```python
from build123d import *

# Parameters (mm, degrees)
F0_W     = 63.5
F0_H     = 127
F0_W_2   = 58.42
F0_H_2   = 121.92
F0_W_3   = 9.398
F0_H_3   = 9.398
F0_W_4   = 12.7
F0_H_4   = 37.084
F0_W_5   = 51.054
F0_H_5   = 21.59
F1_DEPTH = 2.54
F2_DEPTH = 38.1
F3_W     = 58.42
F3_H     = 2.54
F4_DEPTH = 2.54
F6_DEPTH = 12.0904


with BuildPart() as f1:
    # F0 (on Front) → F1 (new body)
    with BuildSketch(Plane.XZ):
        Rectangle(F0_W, F0_H)
        Rectangle(F0_W_2, F0_H_2, mode=Mode.SUBTRACT)
        Rectangle(F0_W_2, F0_H_2)
        with Locations((-19.05, -4.699)):
            Rectangle(F0_W_3, F0_H_3, mode=Mode.SUBTRACT)
        with Locations((19.05, -16.002)):
            Rectangle(F0_W_4, F0_H_4, mode=Mode.SUBTRACT)
        with Locations((0, 40.005)):
            Rectangle(F0_W_5, F0_H_5, mode=Mode.SUBTRACT)
    extrude(amount=-F1_DEPTH)

    # F0 (on Front) → F2 (join)
    with BuildSketch(Plane.XZ):
        Rectangle(F0_W, F0_H)
        Rectangle(F0_W_2, F0_H_2, mode=Mode.SUBTRACT)
    extrude(amount=-F2_DEPTH)

    # F3 (on face) → F4 (join)
    with BuildSketch(Plane(origin=(0, 0, 60.96), x_dir=(1, 0, 0), z_dir=(0, 0, -1))):
        with Locations((0, -36.83)):
            Rectangle(F3_W, F3_H)
    extrude(amount=F4_DEPTH)

    # F5 (on face) → F6 (cut)
    with BuildSketch(Plane.XY.offset(63.5)):
        with BuildLine():
            ThreePointArc((-23.5712, 27.7114), (-18.4912, 22.6314), (-13.4112, 27.7114))
            ThreePointArc((-13.4112, 27.7114), (-18.4912, 32.7914), (-23.5712, 27.7114))
        make_face()
        with BuildLine():
            ThreePointArc((-23.5712, 27.7114), (-18.4912, 32.7914), (-13.4112, 27.7114))
            Line((-13.4112, 27.7114), (-13.4112, 38.1))
            Line((-13.4112, 38.1), (-23.5712, 38.1))
            Line((-23.5712, 38.1), (-23.5712, 27.7114))
        make_face()
    extrude(amount=-F6_DEPTH, mode=Mode.SUBTRACT)


solid = f1.part
```
Geometry: final body of the model. Coordinates: model frame, mm. A direction names the side the tool comes from. Round coordinates to 2 decimals unless told otherwise and drop trailing zeros. Write each loop counter-clockwise with the first axis right and the second up, starting at its lowest first coordinate (ties: lowest second). Pieces come first, ordered by that corner, then holes.
Item 1: Section query B-B (y = 13). Return loops of the section in (x, z), plus the area to 3 significant figures.
Item 2: Mould query, pull axis X, two halves, no side actions, for faces 5 (the face through (8, 37, 58.42)), 6 (the face through (31.75, 19, -1)), 7 (the face through (-31.75, 19, -1)). Classes: +X half, -X half, draft (parallel to the pull), parting line (faces both ways), or undercut.
Item 3: Section query D-D (z = -29). Return loops of the section in (x, y).
Item 4: Pin query (flat end, axial travel): P1, Ø3, axis at x = -19, z = 28.5, coming from the +Y side; P2, Ø12, axis at x = -22, z = -49.5, coming from the -Y side. Return the tip coordinate at first contact, or that it passes through.
Item 5: Section query C-C (x = 23.5). Return loops of the section in (y, z), plus the area to 3 significant figures.
Item 6: Section query A-A (x = -8.5). Return loops of the section in (y, z).
Item 7: Material intervals for L1, parallel to Z at x = 21, y = 4; L2, parallel to X at y = 32, z = -12; L3, parallel to Y at x = -4, z = -34, sorted ascending.
Item 8: Set-up query: faces 1 (the face through (-26, 35.56, 60)), 2 (the face through (-26, 37, 58.42)), 3 (the face through (-19, 1, 0)), 4 (the face through (-13.411, 34, 62)). Return all of +Z, -Z, +X, -X, +Y, -Y with unobstructed straight access to the full face (end or side cutting, diameter ignored); none if empty.
Completed:
1. outline: (-31.75, -63.5) - (31.75, -63.5) - (31.75, 63.5) - (-31.75, 63.5) - close; hole (-29.21, -60.96) - (29.21, -60.96) - (29.21, 60.96) - (-29.21, 60.96) - close
1. area: 942 mm2
2. face 5: undercut
2. face 6: +X half
2. face 7: -X half
3. outline: (-31.75, 0) - (12.7, 0) - (12.7, 2.54) - (-29.21, 2.54) - (-29.21, 38.1) - (-31.75, 38.1) - close; (25.4, 0) - (31.75, 0) - (31.75, 38.1) - (29.21, 38.1) - (29.21, 2.54) - (25.4, 2.54) - close
4. P1: stops at y = 2.54
4. P2: stops at y = 0
5. outline: (0, -63.5) - (38.1, -63.5) - (38.1, -60.96) - (2.54, -60.96) - (2.54, -34.54) - (0, -34.54) - close; (0, 2.54) - (2.54, 2.54) - (2.54, 29.21) - (0, 29.21) - close; (0, 50.8) - (2.54, 50.8) - (2.54, 60.96) - (35.56, 60.96) - (35.56, 58.42) - (38.1, 58.42) - (38.1, 63.5) - (0, 63.5) - close
5. area: 361 mm2
6. outline: (0, -63.5) - (38.1, -63.5) - (38.1, -60.96) - (2.54, -60.96) - (2.54, 29.21) - (0, 29.21) - close; (0, 50.8) - (2.54, 50.8) - (2.54, 60.96) - (35.56, 60.96) - (35.56, 58.42) - (38.1, 58.42) - (38.1, 63.5) - (0, 63.5) - close
7. L1: z = -63.5 to -60.96, 60.96 to 63.5
7. L2: x = -31.75 to -29.21, 29.21 to 31.75
7. L3: y = 0 to 2.54
8. face 1: none
8. face 2: +Y
8. face 3: +Y, -Y
8. face 4: +Z, +Y
